Read the model definition and answer for the solid it produces. Units are mm, in the model's axes. A direction names the side the tool comes from. Coordinates: 2 decimals unless noted, no trailing zeros. Write each loop counter-clockwise with the first axis right and the second up, starting at its lowest first coordinate (ties: lowest second). Pieces come first, ordered by that corner, then holes. Notation, with made-up numbers: (-18, 78.5) -> (-12, 78.5) arc R23 cw to (-12, 113.5) -> close; hole circle Ø7 at (61, 57). An arc over 180 degrees is marked (long way). Write item = value, one per line. Start each with the question number.
1) For a pull along X with two mould halves and no side action, classify faces 1 (the face through (47.5, 1, 2)), 2 (the face through (-20, 22, 5)), 3 (the face through (26.99, -27.15, 1.48)) as released by +X, released by -X, zero draft, split by the parting line, or undercut.
2) A tool of negligible diameter and unlimited length cuts with its end or side. For faces 4 (the face through (-30, 0, 2)), 5 (the face through (1, -47.5, 2)), 6 (the face through (-18.359, -28.797, 3.986)), from which of +Z, -Z, +X, -X, +Y, -Y can it reach the whole face along a straight path? Write none if from no direction.
3) Section A-A (z = 2.25) is taken. Determine the outline of the cut face in (x, y).
4) Section B-B (y = -1.5) is taken. Determine the outline of the cut face in (x, z), plus the area to 3 significant figures.
5) Flat-ended cylindrical pins translate along their axes: pin 1 Ø7 at (x, y) = (25.5, 25) entering from -Z; pin 2 Ø4.5 at (x, y) = (-26, 24.5) entering from -Z. Find the tip coordinate at first contact, or state that the pin passes through.
6) Find the intervals of material crossed by line 1 along X through (y, z) = (-22.5, 4.25); line 2 along Y through (x, z) = (-37.5, 3.9), in increasing order. Write a range as from..to.
from build123d import *

# Parameters (mm, degrees)
SKETCH_1_R          = 1
SKETCH_1_R_2        = 3
EXTRUDE_1_DEPTH     = 5
CUT_EXTRUDE_1_DEPTH = 3


with BuildPart() as part:
    # 草图1 → 凸台-拉伸1 (new body)
    with BuildSketch(Plane.XY):
        with BuildLine():
            Line((-37.5, 47.5), (37.5, 47.5))
            ThreePointArc((37.5, 47.5), (44.571067812, 44.571067812), (47.5, 37.5))
            Line((47.5, 37.5), (47.5, -37.5))
            ThreePointArc((47.5, -37.5), (44.571067812, -44.571067812), (37.5, -47.5))
            Line((37.5, -47.5), (-37.5, -47.5))
            ThreePointArc((-37.5, -47.5), (-44.571067812, -44.571067812), (-47.5, -37.5))
            Line((-47.5, -37.5), (-47.5, 37.5))
            ThreePointArc((-47.5, 37.5), (-44.571067812, 44.571067812), (-37.5, 47.5))
        make_face()
        with Locations((-22.5, 22.5)):
            Circle(SKETCH_1_R, mode=Mode.SUBTRACT)
        with Locations((22.5, 22.5)):
            Circle(SKETCH_1_R, mode=Mode.SUBTRACT)
        with Locations((22.5, -22.5)):
            Circle(SKETCH_1_R, mode=Mode.SUBTRACT)
        with Locations((-22.5, -22.5)):
            Circle(SKETCH_1_R, mode=Mode.SUBTRACT)
        with Locations((37.5, 37.5)):
            Circle(SKETCH_1_R_2, mode=Mode.SUBTRACT)
        with Locations((-37.5, 37.5)):
            Circle(SKETCH_1_R_2, mode=Mode.SUBTRACT)
        with Locations((-37.5, -37.5)):
            Circle(SKETCH_1_R_2, mode=Mode.SUBTRACT)
        with Locations((37.5, -37.5)):
            Circle(SKETCH_1_R_2, mode=Mode.SUBTRACT)
        with BuildLine():
            Line((15.5, 30), (-15.5, 30))
            ThreePointArc((-15.5, 30), (-18.328427125, 28.828427125), (-19.5, 26))
            Line((-19.5, 26), (-19.5, 22.5))
            ThreePointArc((-19.5, 22.5), (-20.378679656, 20.378679656), (-22.5, 19.5))
            Line((-22.5, 19.5), (-26, 19.5))
            ThreePointArc((-26, 19.5), (-28.828427125, 18.328427125), (-30, 15.5))
            Line((-30, 15.5), (-30, -15.5))
            ThreePointArc((-30, -15.5), (-28.828427125, -18.328427125), (-26, -19.5))
            Line((-26, -19.5), (-22.5, -19.5))
            ThreePointArc((-22.5, -19.5), (-20.378679656, -20.378679656), (-19.5, -22.5))
            Line((-19.5, -22.5), (-19.5, -26))
            ThreePointArc((-19.5, -26), (-18.328427125, -28.828427125), (-15.5, -30))
            Line((-15.5, -30), (15.5, -30))
            ThreePointArc((15.5, -30), (18.328427125, -28.828427125), (19.5, -26))
            Line((19.5, -26), (19.5, -22.5))
            ThreePointArc((19.5, -22.5), (20.378679656, -20.378679656), (22.5, -19.5))
            Line((22.5, -19.5), (26, -19.5))
            ThreePointArc((26, -19.5), (28.828427125, -18.328427125), (30, -15.5))
            Line((30, -15.5), (30, 15.5))
            ThreePointArc((30, 15.5), (28.828427125, 18.328427125), (26, 19.5))
            Line((26, 19.5), (22.5, 19.5))
            ThreePointArc((22.5, 19.5), (20.378679656, 20.378679656), (19.5, 22.5))
            Line((19.5, 22.5), (19.5, 26))
            ThreePointArc((19.5, 26), (18.328427125, 28.828427125), (15.5, 30))
        make_face(mode=Mode.SUBTRACT)
    extrude(amount=EXTRUDE_1_DEPTH)

    # 草图2 → 切除-拉伸1 (cut)
    with BuildSketch(Plane(origin=(0, 0, 0), x_dir=(-1, 0, 0), z_dir=(0, 0, -1))):
        with BuildLine():
            Line((20, -30), (-20, -30))
            ThreePointArc((-20, -30), (-27.071067812, -27.071067812), (-30, -20))
            Line((-30, -20), (-30, 20))
            ThreePointArc((-30, 20), (-27.071067812, 27.071067812), (-20, 30))
            Line((-20, 30), (20, 30))
            ThreePointArc((20, 30), (27.071067812, 27.071067812), (30, 20))
            Line((30, 20), (30, -20))
            ThreePointArc((30, -20), (27.071067812, -27.071067812), (20, -30))
        make_face()
    extrude(amount=-CUT_EXTRUDE_1_DEPTH, mode=Mode.SUBTRACT)


solid = part.part
Answer key:
q1.face_1 = released by +X
q1.face_2 = zero draft
q1.face_3 = undercut
q2.face_4 = -Z
q2.face_5 = +Z, -Z, +X, -X, -Y
q2.face_6 = +Z, -Z
q3.outline = (-47.5, -37.5) arc R10 ccw to (-37.5, -47.5) -> (37.5, -47.5) arc R10 ccw to (47.5, -37.5) -> (47.5, 37.5) arc R10 ccw to (37.5, 47.5) -> (-37.5, 47.5) arc R10 ccw to (-47.5, 37.5) -> close; hole circle Ø6 at (-37.5, -37.5); hole circle Ø6 at (-37.5, 37.5); hole (-30, -20) arc R10 ccw to (-20, -30) -> (20, -30) arc R10 ccw to (30, -20) -> (30, 20) arc R10 ccw to (20, 30) -> (-20, 30) arc R10 ccw to (-30, 20) -> close; hole circle Ø6 at (37.5, -37.5); hole circle Ø6 at (37.5, 37.5)
q4.outline = (-47.5, 0) -> (-30, 0) -> (-30, 5) -> (-47.5, 5) -> close; (30, 0) -> (47.5, 0) -> (47.5, 5) -> (30, 5) -> close
q4.area = 175 mm^2
q5.pin_1 = 0
q5.pin_2 = 3
q6.line_1 = -47.5..-23.5, -21.5..-19.5, 19.5..21.5, 23.5..47.5
q6.line_2 = -47.5..-40.5, -34.5..34.5, 40.5..47.5
